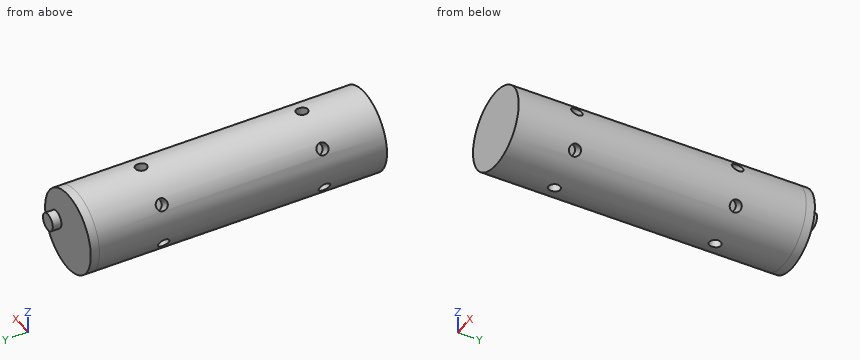
Autodesk Inventor part; units mm, degrees
ref_plane "Work Plane1" through (0, 91.9, 0) normal (0, 1, 0) x (1, 0, 0)
ref_plane "Work Plane3" through (4.9434, 91.9, -15.4641) normal (-0.0831, 0, -0.9965) x (-0.9965, 0, 0.0831)
ref_plane "YZ Plane" through (0, 0, 0) normal (1, 0, 0) x (0, 1, 0)
sketch "Sketch1" plane through (0, 0, 0) normal (0, 1, 0) x (-1, 0, 0)
  circle A0 centre (0, 0) radius 14
  dimension "d0" = 28
extrude "Extrusion1" add sketch "Sketch1" along normal blind 100
ref_plane "Work Plane1" through (0, 91.9, 0) normal (0, 1, 0) x (1, 0, 0)
sketch "Sketch2" plane through (0, 91.9, 0) normal (0, 1, 0) x (1, 0, 0)
  arc A0 (-4.9212, -15.749) -> (7.4582, -14.7182) centre (0, 0) ccw
  line L0 (-4.9212, -15.749) -> (7.4582, -14.7182)
  line L1 (3.8609, -16.2352) -> (3.7603, -15.0261)
  line L2 (1.2685, -15.2336) -> (-1.2229, -15.4411)
  line L3 (-1.1222, -16.6505) -> (-1.2229, -15.4411)
  line L4 (1.7436, -20.9268) -> (4.2347, -20.7192)
  line L5 (4.2347, -20.7192) -> (3.8609, -16.2352)
  line L6 (-1.1222, -16.6505) -> (-0.7484, -21.1346)
  line L7 (-0.7484, -21.1346) -> (1.7436, -20.9268)
  line L8 (8.9092, -10.799) -> (11.1788, -12.1357)
  arc A1 (11.1788, -12.1357) -> (16.4755, -0.8993) centre (0, 0.0004) ccw
  line L9 (11.1788, -12.1357) -> (16.4755, -0.8993)
  line L10 (11.1788, -12.1357) -> (12.7611, -8.7789)
  line L11 (12.7611, -8.7789) -> (17.9297, -11.2153)
  line L12 (17.9297, -11.2153) -> (20.0617, -6.6927)
  line L13 (20.0617, -6.6927) -> (14.893, -4.2562)
  arc A2 (16.0997, 3.6126) -> (9.0172, 13.8181) centre (0, 0) ccw
  line L14 (16.0997, 3.6126) -> (9.0172, 13.8181)
  line L15 (16.0997, 3.6126) -> (13.9839, 6.6614)
  line L16 (13.9839, 6.6614) -> (18.6782, 9.9192)
  line L17 (18.6782, 9.9192) -> (15.8275, 14.0269)
  line L18 (15.8275, 14.0269) -> (11.1332, 10.7691)
  arc A3 (4.9196, 15.7499) -> (-7.4587, 14.7181) centre (0.0003, 0.0003) ccw
  line L19 (4.9196, 15.7499) -> (-7.4587, 14.7181)
  line L20 (4.9196, 15.7499) -> (1.2214, 15.4417)
  line L21 (1.2214, 15.4417) -> (0.7467, 21.1359)
  line L22 (0.7467, 21.1359) -> (-4.236, 20.7206)
  line L23 (-4.236, 20.7206) -> (-3.7613, 15.0263)
  arc A4 (-11.1784, 12.1373) -> (-16.4754, 0.901) centre (0, 0.0009) ccw
  line L24 (-14, 0) -> (-16.4754, 0.901)
  line L25 (-11.1784, 12.1373) -> (-16.4754, 0.901)
  line L26 (-11.1784, 12.1373) -> (-12.7608, 8.7805)
  line L27 (-12.7608, 8.7805) -> (-17.9293, 11.2171)
  line L28 (-17.9293, 11.2171) -> (-20.0613, 6.6944)
  line L29 (-20.0613, 6.6944) -> (-14.8929, 4.2579)
  arc A5 (-16.0997, -3.6126) -> (-9.0172, -13.8181) centre (0, 0) ccw
  line L30 (-9.0172, -13.8181) -> (-16.0997, -3.6126)
  line L31 (-16.0997, -3.6126) -> (-13.9839, -6.6614)
  line L32 (-13.9839, -6.6614) -> (-18.6782, -9.9192)
  line L33 (-18.6782, -9.9192) -> (-15.8275, -14.0269)
  line L34 (-15.8275, -14.0269) -> (-11.1332, -10.7691)
  line L35 (11.1788, -12.1357) -> (-16.4754, 0.901)
  line L36 (16.4755, -0.8993) -> (-11.1784, 12.1373)
  line L37 (-9.0172, -13.8181) -> (16.0997, 3.6126)
  line L38 (-16.0997, -3.6126) -> (9.0172, 13.8181)
  line L39 (-4.9212, -15.749) -> (-7.4587, 14.7181)
  line L40 (7.4582, -14.7182) -> (4.9196, 15.7499)
  line L41 (5.0265, 14.4675) -> (-7.3518, 13.4357)
  dimension "d4" = 2.5
  dimension "d5" = 3.711
  dimension "d6" = 5.714
  dimension "d7" = 5
  dimension "d8" = 3.711
  dimension "d9" = 5.714
  dimension "d10" = 5
  dimension "d11" = 3.711
  dimension "d12" = 5.714
  dimension "d13" = 5
  dimension "d14" = 3.711
  dimension "d15" = 5.714
  dimension "d16" = 5
  dimension "d17" = 3.711
  dimension "d18" = 5.714
  dimension "d19" = 5
  dimension "d20" = 5.258
  dimension "d21" = 0.001
  dimension "d22" = 5.0004
  dimension "d23" = 5.0004
  dimension "d24" = 36.2862
  dimension "d25" = 12.3632
ref_plane "Work Plane2" through (5.0265, 91.9, -14.4675) normal (-0.0831, 0, -0.9965) x (-0.9965, 0, 0.0831)
sketch "Sketch3" plane through (5.0265, 91.9, -14.4675) normal (-0.0831, 0, -0.9965) x (-0.9965, 0, 0.0831)
  line L0 (0, 0) -> (12.421, 0)
  line L1 (20.2109, -91.9) -> (-7.7891, -91.9)
  line L2 (0, -91.9) -> (12.421, -91.9)
  line L3 (12.421, 0) -> (12.421, -91.9) construction
  line L4 (6.2105, 0) -> (6.2105, -15) construction
  circle A0 centre (6.2105, -15) radius 2
  line L5 (6.2105, -91.9) -> (6.2105, -76.9) construction
  circle A1 centre (6.2105, -76.9) radius 2
  point P0 (6.2109, -91.9)
  dimension "d27" = 12.421
  dimension "d28" = 15
  dimension "d29" = 4
  dimension "d30" = 15
  dimension "d31" = 4
ref_plane "Work Plane3" through (4.9434, 91.9, -15.4641) normal (-0.0831, 0, -0.9965) x (-0.9965, 0, 0.0831)
sketch "Sketch4" plane through (4.9434, 91.9, -15.4641) normal (-0.0831, 0, -0.9965) x (-0.9965, 0, 0.0831)
  line L0 (0, 0) -> (12.421, 0)
  line L1 (16.664, -85.9) -> (-11.336, -85.9)
  line L2 (-3.5469, -85.9) -> (12.421, -85.9)
  line L3 (12.421, 0) -> (12.421, -85.9) construction
  line L4 (6.2105, 0) -> (6.2105, -15) construction
  circle A0 centre (6.2105, -15) radius 2
  line L5 (6.2105, -85.9) -> (6.2105, -70.9) construction
  circle A1 centre (6.2105, -70.9) radius 2
  line L6 (6.2105, -76.9) -> (6.2105, -70.9) construction
  point P0 (6.2109, -91.9)
  point P1 (6.2109, -91.9)
  dimension "d33" = 12.421
  dimension "d34" = 15
  dimension "d35" = 4
  dimension "d36" = 15
  dimension "d37" = 4
  dimension "d43" = 6
extrude "Extrusion2" cut sketch "Sketch4" against normal blind 5.5
pattern_circular "Circular Pattern1" count 6 over 360 about axis through (0, -10, 0) along (0, 1, 0) of "Extrusion2"
sketch "Sketch5" plane through (0, 100, 0) normal (0, 1, 0) x (1, 0, 0)
  line L0 (0, 0) -> (14, 0) construction
  circle A0 centre (0, 0) radius 14 construction
  line L1 (0, 0) -> (7, 0) construction
  circle A1 centre (7, 0) radius 3
  dimension "d44" = 6
extrude "Extrusion3" add sketch "Sketch5" along normal blind 6
sketch "Sketch6" plane through (0, 100, 0) normal (0, 1, 0) x (1, 0, 0)
  circle A0 centre (0, 0) radius 14
extrude "Extrusion4" add sketch "Sketch6" along normal blind 3
properties part number "Grip Base"
CAD build for the part. Positions are in the model's coordinates, mm. Round coordinates to 2 decimals unless told otherwise and drop trailing zeros. Loops run counter-clockwise (first coordinate to the right, second up) from the corner with the lowest first, then second, coordinate; pieces in that order, holes last. Notation, with made-up numbers: M 27,74 L 46,74 A24 ccw 46,86 Z; hole C 11.5,-30.75 d2. An arc over 180 degrees is marked long. Use a Markdown table: item, result. Add a question column.
(1) Cut at B-B (y = 29). Give the cut face in (x, z), and give its area (3 significant figures).
(2) Flat gauge pins, fed straight in: pin 1 (10 mm diameter, centred on y = 23, z = 8.5, fed in from -X); pin 2 (3 mm diameter, centred on x = -2, y = 42, fed in from +Z); pin 3 (4 mm diameter, centred on y = 60.5, z = 9.5, fed in from +X). Where does each tip first touch, or does it go through?
(3) Drill centre lines: line 1 (Y direction, x = 7.5, z = -7); line 2 (Y direction, x = 8.75, z = 8.25); line 3 (Z direction, x = -6.25, y = 44.5). Where is each one in solid material? Low to high.
(4) Cut at A-A (z = 0). Give the cut face in (x, y).
Geometry says:
| question | item | result |
|---|---|---|
| 1 | outline | C 0,0 d28 |
| 1 | area | 616 mm² |
| 2 | pin 1 | stops at x = -13.56 |
| 2 | pin 2 | stops at z = 13.99 |
| 2 | pin 3 | stops at x = 11.82 |
| 3 | line 1 | y = 0 to 19.65, 22.35 to 75.55, 78.25 to 103 |
| 3 | line 2 | y = 0 to 103 |
| 3 | line 3 | z = -12.53 to 12.53 |
| 4 | outline | M -14,0 L 14,0 L 14,103 L 10,103 L 10,106 L 4,106 L 4,103 L -14,103 Z |
